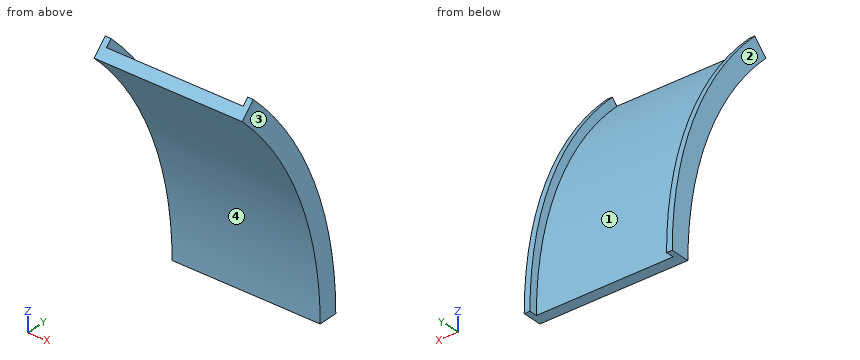
```python
from build123d import *

# Parameters (mm, degrees)
REVOLVE2_ANGLE = 45


with BuildPart() as part:
    # Sketch1 → Revolve2 (revolve)
    with BuildSketch(Plane.XY):
        Polygon((0, 0), (25, 0), (25, -35.236081748), (625, -35.236081748), (625, 0), (650, 0), (650, -85.236081748), (0, -85.236081748), align=None)
    revolve(axis=Axis((0, -1535.236081748, 0), (1, 0, 0)), revolution_arc=REVOLVE2_ANGLE)


solid = part.part
```
The model under review builds one solid part; all positions refer to its coordinate system, in mm. Face numbers are marked on the shaded views. Round coordinates to 2 decimals unless told otherwise and drop trailing zeros. Write each loop counter-clockwise with the first axis right and the second up, starting at its lowest first coordinate (ties: lowest second). Pieces come first, ordered by that corner, then holes. Notation, with made-up numbers: (-28, -15) - (4, -15) arc R34 cw to (4, 17) - close; hole circle Ø8 at (41, 21.5). An arc over 180 degrees is marked (long way). Answer as CSV lines item,"result". Start each with the question number.
(1) To check wall thickness, follow line 1 (Y direction, x = 587, z = 207.5); line 2 (Z direction, x = 49, y = -401); line 3 (Y direction, x = 455.5, z = 661). State the ranges of each line that lie inside material, in increasing order.
(2) For pin 1 Ø4 at (x, z) = (482.5, 477.5) entering from +Y; pin 2 Ø5 at (x, y) = (325, -298.5) entering from -Z; pin 3 Ø1.5 at (x, y) = (367.5, -384.5) entering from -Z, all flat-tipped, find the tip position at first contact; note any pin that passes through.
(3) We need section B-B on y = -250. State the section outline as (x, z) points.
(4) We need section A-A on z = 836. State the section outline as (x, y) points.
(5) Draft analysis for pull direction X (two halves, no side actions). For the marked faces 1, 2, 3 and 4, state which applies: pulls with the +X half, pulls with the -X half, needs draft (parallel to the pull), parting line crosses it, or undercut.
(6) We need section C-C on x = 69.5. State the section outline as (y, z) points.
Worked answers:
1,line 1,"-100.16 to -49.66"
1,line 2,"903.33 to 981.58"
1,line 3,"-244.66 to -188.73"
2,pin 1,"y = -112.6"
2,pin 2,"z = 752.86"
2,pin 3,"z = 881.24"
3,outline,"(0, 671.32) - (650, 671.32) - (650, 839.71) - (625, 839.71) - (625, 773.41) - (25, 773.41) - (25, 839.71) - (0, 839.71) - close"
4,outline,"(0, -350.5) - (650, -350.5) - (650, -247.58) - (625, -247.58) - (625, -289.8) - (25, -289.8) - (25, -247.58) - (0, -247.58) - close"
5,face 1,"undercut"
5,face 2,"pulls with the -X half"
5,face 3,"pulls with the +X half"
5,face 4,"needs draft"
6,outline,"(-509.93, 1025.3) arc R1450 cw to (-85.24, 0) - (-35.24, 0) arc R1500 ccw to (-474.58, 1060.66) - close"
